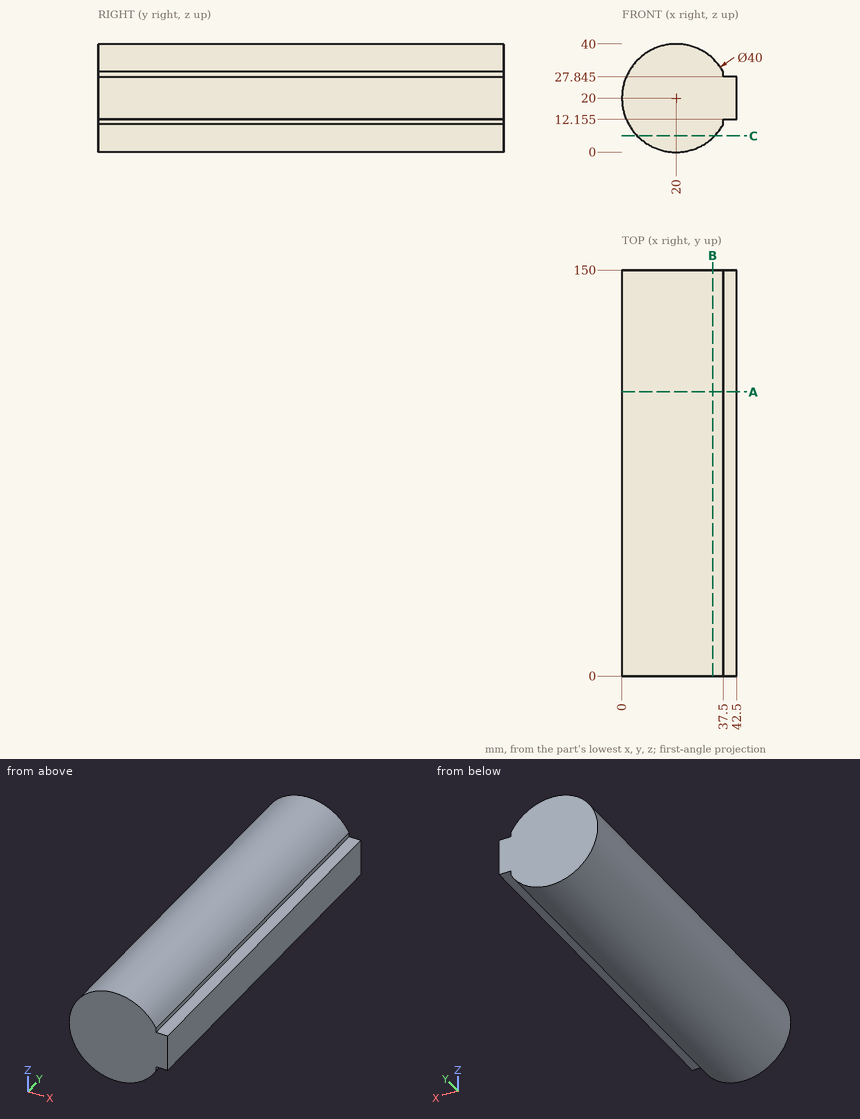
Input: dimensioned drawing with shaded views. Units: mm. Origin: part minimum x, y, z. Give positions to 0.01 mm unless a question says otherwise; leave off trailing zeros. Write each loop counter-clockwise with the first axis right and the second up, starting at its lowest first coordinate (ties: lowest second). Pieces come first, ordered by that corner, then holes.
1. Material intervals for line 1 along X through (y, z) = (42, 20.5); line 2 along X through (y, z) = (81.5, 14); line 3 along Z through (x, y) = (3, 78) (1 decimal), sorted ascending.
2. First-contact query: pin 1 (5.5 mm diameter, centred on x = 39.5, y = 104.5, fed in from +Z); pin 2 (2 mm diameter, centred on y = 52.5, z = 11, fed in from +X); pin 3 (5 mm diameter, centred on x = 25.5, y = 40, fed in from +Z). Flat tips, straight axial feed; report the tip coordinate or a pass-through.
3. Section query C-C (z = 6). Return the cut outline in (x, y).
4. Section query B-B (x = 33.5). Return the cut outline in (y, z), then the cut area to 3 significant figures.
5. Section query A-A (y = 105). Return the cut outline in (x, z) (1 decimal).
Output values:
1. line 1: x = 0.01 to 42.5
1. line 2: x = 0.92 to 42.5
1. line 3: z = 9.5 to 30.5
2. pin 1: stops at z = 30.93
2. pin 2: stops at x = 37.5
2. pin 3: stops at z = 39.77
3. outline: (5.72, 0) - (34.28, 0) - (34.28, 150) - (5.72, 150) - close
4. outline: (0, 5.24) - (150, 5.24) - (150, 34.76) - (0, 34.76) - close
4. area: 4,430 mm2
5. outline: (37.5, 10.3) - (37.5, 12.2) - (42.5, 12.2) - (42.5, 27.8) - (37.5, 27.8) - (37.5, 29.7) arc R20 ccw (long way) to start
